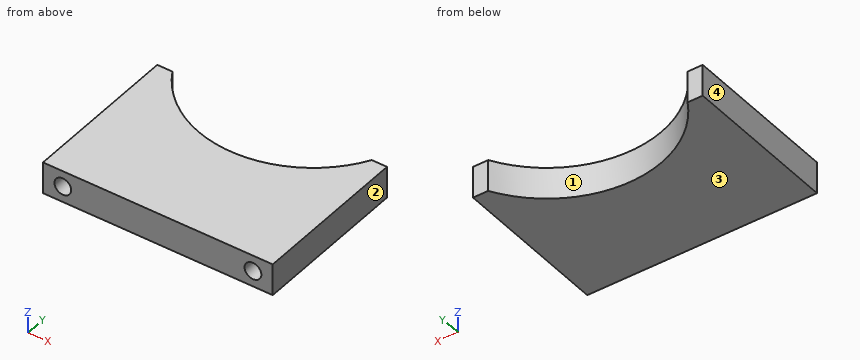
from build123d import *

# Parameters (mm, degrees)
BOSS_EXTRUDE1_DEPTH = 6.35
SKETCH2_R           = 3.3655
CUT_EXTRUDE1_DEPTH  = 12.7


with BuildPart() as part:
    # Sketch1 → Boss-Extrude1 (new body, symmetric)
    with BuildSketch(Plane.XY):
        with BuildLine():
            Line((-46.0375, 63.5), (-39.960878447, 63.5))
            ThreePointArc((-39.960878447, 63.5), (0, 40.3225), (39.960878447, 63.5))
            Line((39.960878447, 63.5), (46.0375, 63.5))
            Line((46.0375, 63.5), (46.0375, 0))
            Line((46.0375, 0), (-46.0375, 0))
            Line((-46.0375, 0), (-46.0375, 63.5))
        make_face()
    extrude(amount=BOSS_EXTRUDE1_DEPTH, both=True)

    # Sketch2 → Cut-Extrude1 (cut)
    with BuildSketch(Plane.XZ):
        with Locations((-38.1, 0)):
            Circle(SKETCH2_R)
        with Locations((38.1, 0)):
            Circle(SKETCH2_R)
    extrude(amount=-CUT_EXTRUDE1_DEPTH, mode=Mode.SUBTRACT)


solid = part.part
Read the model definition and answer for the solid it produces. Units are mm, in the model's axes. Face numbers are marked on the shaded views. Coordinates: 2 decimals unless noted, no trailing zeros. Order: outer loops, then holes, each group sorted by start corner. A loop starts at its lowest first (then second) coordinate and runs counter-clockwise, first axis right, second up. Notation, with made-up numbers: M -6,8 L 27,8 A29 cw 27,35 Z; hole C 45.5,28 d7. An arc over 180 degrees is marked long. Put each result on its own line as item: value. Start each with the question number.
Item 1: Section C-C, the plane x = -38.1 is taken. Determine the outline of the cut face in (y, z), plus the area to 3 significant figures.
Item 2: Given pin 1 Ø4 at (x, z) = (30, -4.5) entering from -Y; pin 2 Ø5 at (x, z) = (-18.5, 2.5) entering from +Y; pin 3 Ø3.5 at (x, z) = (-39.5, 0.5) entering from -Y, each flat-ended and moving along its own axis, determine where each tip first touches the part or whether it passes through.
Item 3: Section B-B, the plane y = 56 is taken. Determine the outline of the cut face in (x, z).
Item 4: Section D-D, the plane z = 4.5 is taken. Determine the outline of the cut face in (x, y) (1 decimal).
Item 5: The mould has two halves that part along X. Classify the marked faces 1, 2, 3 and 4: +X half, -X half, draft (parallel to the pull), parting line (faces both ways), or undercut.
Item 6: Section A-A, the plane z = 0 is taken. Determine the outline of the cut face in (x, y) (1 decimal).
Item 7: Consider probe 1 along Z at (x, y) = (38, 3); probe 2 along Z at (x, y) = (-41, 4); probe 3 along X at (y, z) = (49.5, 0.25). Determine where each line is inside the solid, lowest interval first. Write a range as [from, to].
Computed:
1. outline: M 0,-6.35 L 60.52,-6.35 L 60.52,6.35 L 0,6.35 L 0,3.37 L 12.7,3.37 L 12.7,-3.37 L 0,-3.37 Z
1. area: 683 mm2
2. pin 1: stops at y = 0
2. pin 2: stops at y = 45.39
2. pin 3: stops at y = 12.7
3. outline: M -46.04,-6.35 L -34.61,-6.35 L -34.61,6.35 L -46.04,6.35 Z; M 34.61,-6.35 L 46.04,-6.35 L 46.04,6.35 L 34.61,6.35 Z
4. outline: M -46,0 L 46,0 L 46,63.5 L 40,63.5 A46 cw -40,63.5 L -46,63.5 Z
5. face 1: undercut
5. face 2: +X half
5. face 3: draft
5. face 4: -X half
6. outline: M -46,0 L -41.5,0 L -41.5,12.7 L -34.7,12.7 L -34.7,0 L 34.7,0 L 34.7,12.7 L 41.5,12.7 L 41.5,0 L 46,0 L 46,63.5 L 40,63.5 A46 cw -40,63.5 L -46,63.5 Z
7. probe 1: z = [-6.35, -3.36], [3.36, 6.35]
7. probe 2: z = [-6.35, -1.71], [1.71, 6.35]
7. probe 3: x = [-46.04, -27.58], [27.58, 46.04]
